Verification items for the finished model (mm, model axes). Give positions to 0.01 mm unless a question says otherwise; leave off trailing zeros. Write each loop counter-clockwise with the first axis right and the second up, starting at its lowest first coordinate (ties: lowest second). Pieces come first, ordered by that corner, then holes. Notation, with made-up numbers: M 43.5,4 L 96.5,4 A18 ccw 96.5,21 Z; hole C 52.25,-18 d9. An arc over 180 degrees is marked long. Answer as a JSON object with one key per item and string values.
```python
from build123d import *

# Parameters (mm, degrees)
SKETCH_W  = 180
SKETCH_H  = 70
SKETCH_R  = 4
PAD_DEPTH = 10
FILLET_R  = 10


with BuildPart() as part:
    # Sketch → Pad (new body)
    with BuildSketch(Plane.XY):
        with Locations((60, 25)):
            Rectangle(SKETCH_W, SKETCH_H)
        with Locations((-15, 45)):
            Circle(SKETCH_R, mode=Mode.SUBTRACT)
        with Locations((135, 45)):
            Circle(SKETCH_R, mode=Mode.SUBTRACT)
        with Locations((-15, 5)):
            Circle(SKETCH_R, mode=Mode.SUBTRACT)
        with Locations((135, 5)):
            Circle(SKETCH_R, mode=Mode.SUBTRACT)
        with Locations((12, 45)):
            Circle(SKETCH_R, mode=Mode.SUBTRACT)
        with Locations((108, 45)):
            Circle(SKETCH_R, mode=Mode.SUBTRACT)
        with Locations((12, 15)):
            Circle(SKETCH_R, mode=Mode.SUBTRACT)
        with Locations((108, 15)):
            Circle(SKETCH_R, mode=Mode.SUBTRACT)
    extrude(amount=PAD_DEPTH)

    # Fillet
    fillet_edges = [part.edges().sort_by_distance(p)[0] for p in [
        (-30, -10, 5),
        (-30, 60, 5),
        (150, -10, 5),
        (150, 60, 5),
    ]]
    fillet(fillet_edges, radius=FILLET_R)


solid = part.part
```
1) Section check B-B on y = 45. Record the boundary of the cut face in (x, z).
Completed:
{"outline": "M -30,0 L -19,0 L -19,10 L -30,10 Z; M -11,0 L 8,0 L 8,10 L -11,10 Z; M 16,0 L 104,0 L 104,10 L 16,10 Z; M 112,0 L 131,0 L 131,10 L 112,10 Z; M 139,0 L 150,0 L 150,10 L 139,10 Z"}
2) Section check C-C on y = 15. Record the boundary of the cut face in (x, z).
Completed:
{"outline": "M -30,0 L 8,0 L 8,10 L -30,10 Z; M 16,0 L 104,0 L 104,10 L 16,10 Z; M 112,0 L 150,0 L 150,10 L 112,10 Z"}
3) Section check D-D on z = 8. Count the separate pieces of the cut face and the enclosed holes in it, and give its area (3 significant figures).
Completed:
{"separate pieces": "1", "enclosed holes": "8", "area": "12,100 mm2"}
4) Thickness scan on L1, parallel to Y at x = 12, z = 4.25; L2, parallel to X at y = 15.5, z = 5; L3, parallel to Y at x = 135, z = 3.25. Record the ranges inside material, lowest first.
Completed:
{"L1": "y = -10 to 11, 19 to 41, 49 to 60", "L2": "x = -30 to 8.03, 15.97 to 104.03, 111.97 to 150", "L3": "y = -10 to 1, 9 to 41, 49 to 60"}
5) Section check A-A on x = 12. Record the boundary of the cut face in (y, z), and give its area (3 significant figures).
Completed:
{"outline": "M -10,0 L 11,0 L 11,10 L -10,10 Z; M 19,0 L 41,0 L 41,10 L 19,10 Z; M 49,0 L 60,0 L 60,10 L 49,10 Z", "area": "540 mm2"}
6) Release check for a two-part mould opening along X. For faces 1 (the face through (-30, 25, 5)), 2 (the face through (59, 25, 0)), 3 (the face through (150, 25, 5)), 4 (the face through (8.8, 42.6, 4.9)) record: pulls with the +X half, pulls with the -X half, needs draft (parallel to the pull), parting line crosses it, or undercut.
Completed:
{"face 1": "pulls with the -X half", "face 2": "needs draft", "face 3": "pulls with the +X half", "face 4": "undercut"}
